```python
from build123d import *


with BuildPart() as f1:
    # F0 (on Front) → F1 (revolve)
    with BuildSketch(Plane.XZ):
        with BuildLine():
            Line((0, 4.737021), (0, 0))
            Line((0, 0), (27.94, 0))
            ThreePointArc((27.94, 0), (27.254253, 1.378937), (26.139495, 2.441496))
            ThreePointArc((26.139495, 2.441496), (22.802874, 3.991977), (19.1516, 4.445))
            Line((19.1516, 4.445), (19.1516, 4.826))
            Line((19.1516, 4.826), (2.957049, 4.9657))
            Line((2.957049, 4.9657), (2.159, 4.4069))
            Line((2.159, 4.4069), (1.27, 4.4069))
            Line((1.27, 4.4069), (1.27, 5.0038))
            Line((1.27, 5.0038), (0.381, 5.0038))
            Line((0.381, 5.0038), (0, 4.737021))
        make_face()
    revolve(axis=Axis((19.091603, 0, 0), (1, 0, 0)))


solid = f1.part
```
CAD build for the part. Positions are in the model's coordinates, mm. A direction names the side the tool comes from. Coordinates: 2 decimals unless noted, no trailing zeros. Order: outer loops, then holes, each group sorted by start corner. A loop starts at its lowest first (then second) coordinate and runs counter-clockwise, first axis right, second up. Notation, with made-up numbers: (46, 76.5) - (87, 76.5) arc R13 ccw to (87, 95.5) - close; hole circle Ø10 at (86.5, -37). An arc over 180 degrees is marked (long way). Use a Markdown table: item, result. Add a question column.
(1) Which spindle directions (+Z, -Z, +X, -X, +Y, -Y) get a long thin tool onto all of the face, cutting with end or side? Do faces 1 (the face through (1.71, 4.3, -0.96)), 2 (the face through (10.94, 4.78, -1.06)), 3 (the face through (0, 0, 0)). Say none if no direction does.
(2) Saw through at B-B (x = 11.75). Give the cut face in (y, z).
(3) Drill centre lines: line 1 along Y through (x, z) = (25.25, 0.5); line 2 along Y through (x, z) = (19, 3.5); line 3 along Z through (x, y) = (19, 0). Where is each one in solid material? Low to high. Write a range as [from, to].
(4) Saw through at A-A (x = 16.5). Give the cut face in (y, z).
(5) Flat gauge pins, fed straight in: pin 1 (2 mm diameter, centred on x = 11.5, z = 4, fed in from -Y); pin 2 (2 mm diameter, centred on x = 8, z = 0, fed in from +Y); pin 3 (1 mm diameter, centred on x = 21.5, y = 0, fed in from -Z). Where does each tip first touch, or does it go through?
Solved:
| question | item | result |
|---|---|---|
| 1 | face 1 | none |
| 1 | face 2 | +X |
| 1 | face 3 | +Z, -Z, -X, +Y, -Y |
| 2 | outline | circle Ø9.78 at (0, 0) |
| 3 | line 1 | y = [-2.94, 2.94] |
| 3 | line 2 | y = [-3.32, 3.32] |
| 3 | line 3 | z = [-4.83, 4.83] |
| 4 | outline | circle Ø9.7 at (0, 0) |
| 5 | pin 1 | stops at y = -3.86 |
| 5 | pin 2 | stops at y = 4.93 |
| 5 | pin 3 | stops at z = -4.36 |
